Here's how the part is built. I have some questions about the finished solid (model axes, mm). A direction names the side the tool comes from. Coordinates: 2 decimals unless noted, no trailing zeros. Order: outer loops, then holes, each group sorted by start corner. A loop starts at its lowest first (then second) coordinate and runs counter-clockwise, first axis right, second up. Notation, with made-up numbers: (-36, -39.75) - (23, -39.75) arc R16 ccw to (23, -11.75) - close; hole circle Ø8 at (20, -15). An arc over 180 degrees is marked (long way). Answer as CSV lines item,"result". Start each with the question number.
Q1. Suppose I cut it at B-B (x = 18.5). Please give me the cut outline in (y, z), then the cut area to 3 significant figures.
Q2. For pin 1 Ø1.5 at (y, z) = (16, 10.5) entering from +X; pin 2 Ø1.5 at (x, y) = (27, 10.5) entering from +Z; pin 3 Ø1 at (x, z) = (27, 14) entering from +Y; pin 4 Ø2 at (y, z) = (5.5, 8) entering from -X, each with a flat end and sliding along its axis, tell me the tip position at first contact or that it passes through.
Q3. I need wall thicknesses on line 1 (X direction, y = -19.5, z = 8); line 2 (Z direction, x = -21, y = 5.5); line 3 (X direction, y = 21, z = 3.75). Which ranges of each line are inside material? Lowest first, please.
Q4. Suppose I cut it at A-A (y = -9.5). Please give me the cut outline in (x, z).
Q5. For faces 1 (the face through (25, -6, 8)), 2 (the face through (15, 25, 2)), 3 (the face through (27, -5, 14)), which set-ups out of +Z, -Z, +X, -X, +Y, -Y let a thin tool reach every point of the face, with its end or its side?
Q6. Suppose I cut it at D-D (y = 0). Please give me the cut outline in (x, z), then the cut area to 3 significant figures.
Q7. Suppose I cut it at C-C (z = 8.25). Please give me the cut outline in (x, y).
from build123d import *

# Parameters (mm, degrees)
F1_DEPTH = 5
F2_W     = 5
F2_H     = 50
F3_DEPTH = 4
F4_W     = 5
F4_H     = 20
F5_DEPTH = 10.5
F6_R     = 3


with BuildPart() as f1:
    # F0 (on Top) → F1 (new body)
    with BuildSketch(Plane.XY):
        with BuildLine():
            Line((30, 25), (0, 25))
            ThreePointArc((0, 25), (-25, 0), (0, -25))
            Line((0, -25), (30, -25))
            Line((30, -25), (30, 25))
        make_face()
    extrude(amount=F1_DEPTH)

    # F2 (on face) → F3 (join)
    with BuildSketch(Plane.XY.offset(5)):
        with Locations((27.5, 0)):
            Rectangle(F2_W, F2_H)
    extrude(amount=F3_DEPTH)

    # F4 (on face) → F5 (join)
    with BuildSketch(Plane.XY.offset(5)):
        with Locations((27.5, -15)):
            Rectangle(F4_W, F4_H)
    extrude(amount=F5_DEPTH)

    # F6
    f6_edges = [f1.edges().sort_by_distance(p)[0] for p in [
        (27.5, -5, 9),
        (25, -15, 15.5),
    ]]
    fillet(f6_edges, radius=F6_R)


solid = f1.part
Here are the results:
1,outline,"(-25, 0) - (25, 0) - (25, 5) - (-25, 5) - close"
1,area,"250 mm²"
2,pin 1,"passes through"
2,pin 2,"stops at z = 9"
2,pin 3,"stops at y = -5"
2,pin 4,"stops at x = 25"
3,line 1,"x = 25 to 30"
3,line 2,"z = 0 to 5"
3,line 3,"x = -13.56 to 30"
4,outline,"(-23.12, 0) - (30, 0) - (30, 15.5) - (28, 15.5) arc R3 ccw to (25, 12.5) - (25, 5) - (-23.12, 5) - close"
5,face 1,"+Z, -X, +Y, -Y"
5,face 2,"+Z, -Z, +X, -X, +Y"
5,face 3,"+Z, +X, -X, +Y"
6,outline,"(-25, 0) - (30, 0) - (30, 9) - (25, 9) - (25, 5) - (-25, 5) - close"
6,area,"295 mm²"
7,outline,"(25, -25) - (30, -25) - (30, 25) - (25, 25) - close"
